For this review, take the finished solid that the model builds, in its own axes (mm). Give positions to 0.01 mm unless a question says otherwise; leave off trailing zeros. Order: outer loops, then holes, each group sorted by start corner. A loop starts at its lowest first (then second) coordinate and runs counter-clockwise, first axis right, second up. Notation, with made-up numbers: M -26,31 L -15,31 A27 ccw -15,53 Z; hole C -19.75,73 d1. An arc over 180 degrees is marked long. Answer as CSV lines item,"result". Start each with the question number.
1. For line 1 along X through (y, z) = (-6, 38); line 2 along Z through (x, y) = (0, -13) (3 decimals); line 3 along X through (y, z) = (-18, 71.5), list the stretches that pass through material, from the lowest coordinate up.
2. We need section A-A, the plane x = 0. Give the boundary of the cut face in (y, z) (3 decimals).
3. We need section B-B, the plane z = 38.1. Give the boundary of the cut face in (x, y) (3 decimals).
from build123d import *

# Parameters (mm, degrees)
F0_W        = 58.722935617
F0_H        = 47.8591956198
F1_DEPTH    = 76.2
F2_R        = 5.08
F3_T1_DEPTH = 73.962935617
F5_D        = 6.35


# Not quite as in the source:
# - a fillet or chamfer that OpenCascade refuses, or shapes differently, is made with other operations: its cross-section is extruded or revolved along the edge and cut away or added


with BuildPart() as f1:
    # F0 (on Top) → F1 (new body)
    with BuildSketch(Plane.XY):
        Rectangle(F0_W, F0_H)
    extrude(amount=F1_DEPTH)

    # F2
    f2_edges = [f1.edges().sort_by_distance(p)[0] for p in [
        (29.361468, 23.929598, 38.1),
        (0, 23.929598, 76.2),
        (-29.361468, 23.929598, 38.1),
        (0, 23.929598, 0),
        (29.361468, 0, 76.2),
        (29.361468, -23.929598, 38.1),
        (29.361468, 0, 0),
        (-29.361468, 0, 76.2),
        (-29.361468, -23.929598, 38.1),
        (-29.361468, 0, 0),
    ]]
    fillet(f2_edges, radius=F2_R)

    # F3: fillet of radius 5.08 on 4 edges, made by hand

    # F3_s2 → F3_t1 (cut)
    with BuildSketch(Plane.YZ.offset(-36.9814678085)):
        with BuildLine():
            ThreePointArc((-18.8495978099, 0), (-22.4417002583, 1.4878975516), (-23.9295978099, 5.08))
            Line((-23.9295978099, 5.08), (-23.9295978099, 0))
            Line((-23.9295978099, 0), (-18.8495978099, 0))
        make_face()
        with BuildLine():
            ThreePointArc((-18.8495978099, 76.2), (-22.4417002583, 74.7121024484), (-23.9295978099, 71.12))
            Line((-23.9295978099, 71.12), (-23.9295978099, 76.2))
            Line((-23.9295978099, 76.2), (-18.8495978099, 76.2))
        make_face()
    extrude(amount=F3_T1_DEPTH, mode=Mode.SUBTRACT)

    # F5 (through all)
    with Locations(Plane.XZ.offset(23.9295978099)):
        with Locations((0, 38.1)):
            Hole(F5_D / 2)


solid = f1.part
Result set:
1,line 1,"-29.36 to -3.17, 3.17 to 29.36"
1,line 2,"0 to 34.925, 41.275 to 76.2"
1,line 3,"-29.35 to 29.35"
2,outline,"M -23.93,5.08 A5.08 ccw -18.85,0 L 18.85,0 A5.08 ccw 23.93,5.08 L 23.93,34.925 L -23.93,34.925 Z; M -23.93,41.275 L 23.93,41.275 L 23.93,71.12 A5.08 ccw 18.85,76.2 L -18.85,76.2 A5.08 ccw -23.93,71.12 Z"
3,outline,"M -29.361,-18.85 A5.08 ccw -24.281,-23.93 L -3.175,-23.93 L -3.175,23.93 L -24.281,23.93 A5.08 ccw -29.361,18.85 Z; M 3.175,-23.93 L 24.281,-23.93 A5.08 ccw 29.361,-18.85 L 29.361,18.85 A5.08 ccw 24.281,23.93 L 3.175,23.93 Z"
